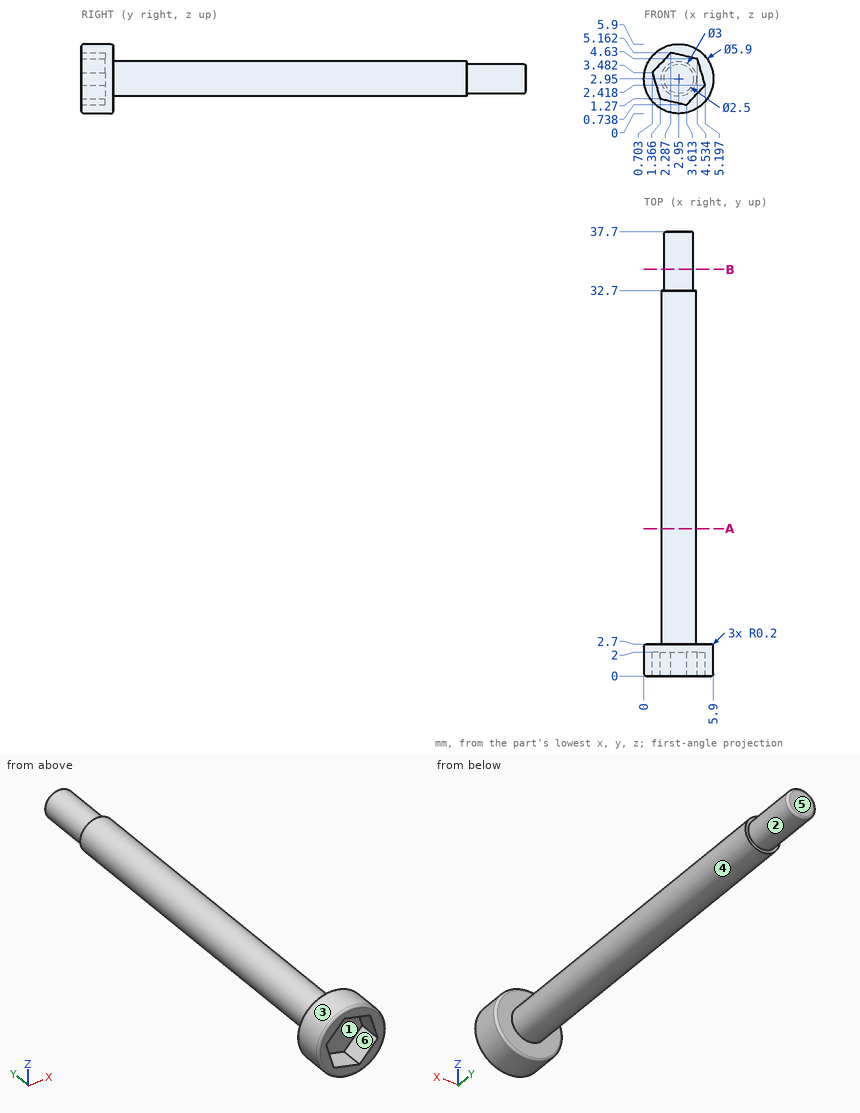
Could you check a few things on this drawing? It's one solid part, dimensions in mm from its lowest x, y, z. A direction names the side the tool comes from. Round coordinates to 2 decimals unless told otherwise and drop trailing zeros. Write each loop counter-clockwise with the first axis right and the second up, starting at its lowest first coordinate (ties: lowest second). Pieces come first, ordered by that corner, then holes. Notation, with made-up numbers: M 28.5,89 L 81.5,89 A21 cw 81.5,120 Z; hole C -21.5,30.25 d7. An arc over 180 degrees is marked long. Answer as CSV lines item,"result". Start each with the question number.
1. I need wall thicknesses on probe 1 along Y at (x, z) = (3.45, 1.7); probe 2 along Y at (x, z) = (3.85, 0.8); probe 3 along Z at (x, y) = (2.4, 13) (1 decimal). Which ranges of each line are inside material? Lowest first, please.
2. I'm going to push flat-ended pins straight in: pin 1 Ø1 at (y, z) = (29.5, 3.5) entering from -X; pin 2 Ø3.5 at (x, z) = (3, 3.5) entering from -Y; pin 3 Ø1 at (x, y) = (2, 18.5) entering from +Z. Where does each tip first touch, or does it pass through?
3. On a 3-axis mill with a long thin cutter (end or side, diameter ignored), from which of +Z, -Z, +X, -X, +Y, -Y can I reach the whole of each face in a straight line? I mean the marked faces 1, 2 and 3. Say none if no direction works.
4. Suppose I cut it at A-A on y = 12.5. Write out the boundary of the cut face in (x, z).
5. Suppose I cut it at B-B on y = 34.5. Write out the boundary of the cut face in (x, z).
6. Thinking about a two-plate mould opening in Z: for the marked faces 4, 5 and 6, which applies, released by +Z, released by -Z, zero draft, split by the parting line, or undercut?
Check result:
1,probe 1,"y = 2 to 32.7"
1,probe 2,"y = 0 to 2.7"
1,probe 3,"z = 1.6 to 4.3"
2,pin 1,"stops at x = 1.45"
2,pin 2,"stops at y = 0"
2,pin 3,"stops at z = 4.38"
3,face 1,"-Y"
3,face 2,"+Y"
3,face 3,"+Y, -Y"
4,outline,"C 2.95,2.95 d3"
5,outline,"C 2.95,2.95 d2.5"
6,face 4,"split by the parting line"
6,face 5,"zero draft"
6,face 6,"undercut"
